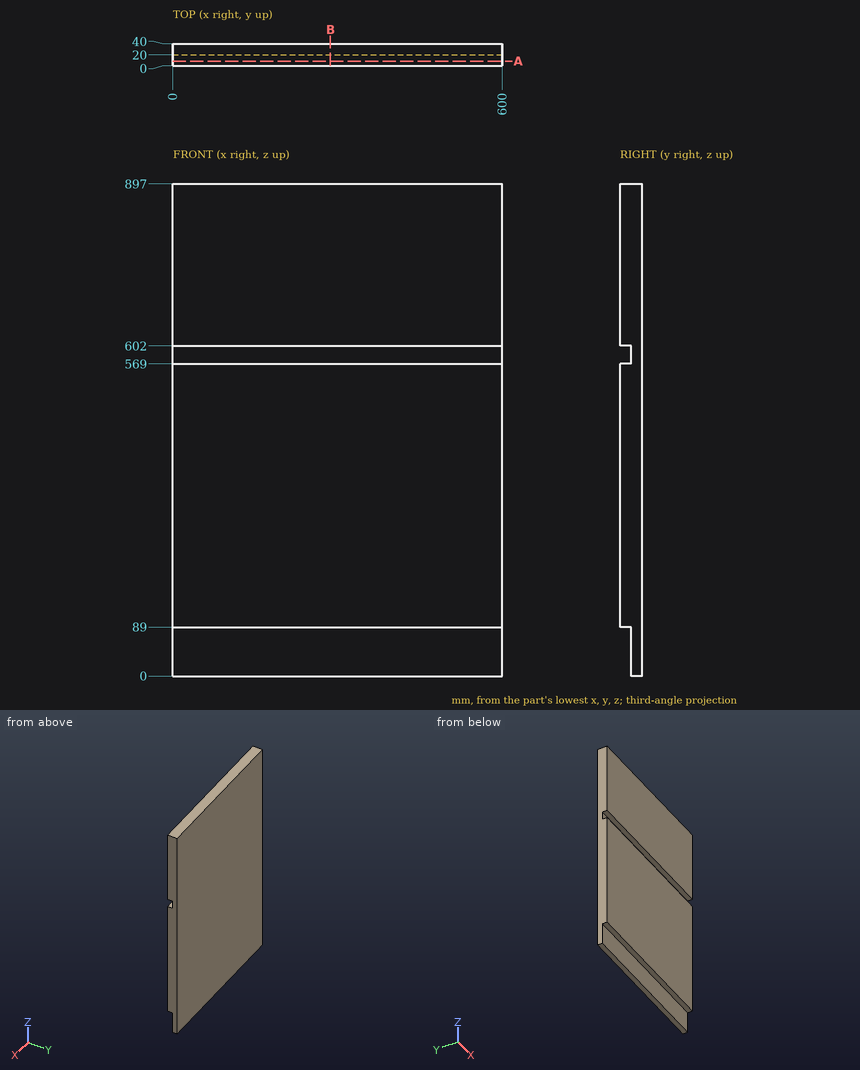
Print and shaded views of the part. All mm, measured from the part's lowest x, y and z. Round coordinates to 2 decimals unless told otherwise and drop trailing zeros. Write each loop counter-clockwise with the first axis right and the second up, starting at its lowest first coordinate (ties: lowest second). Pieces come first, ordered by that corner, then holes.
(1) Slice it at A-A, the plane y = 9. Write the cut outline in (x, z), and give its area (3 significant figures).
(2) Drop a flat-ended pin along its axis: P1, Ø10, axis at x = 443.5, z = 591.5, coming from the -Y side. Give the stop position or say it passes through.
(3) Slice it at B-B, the plane x = 287. Write the cut outline in (y, z).
(4) Probe line 1 along Z through (x, y) = (398.5, 19); line 2 along Y through (x, z) = (218, 83). List the from-to ranges inside material, lowest first.
From the geometry:
1. outline: (0, 89) - (600, 89) - (600, 569) - (0, 569) - close; (0, 602) - (600, 602) - (600, 897) - (0, 897) - close
1. area: 465,000 mm2
2. P1: stops at y = 20
3. outline: (0, 89) - (20, 89) - (20, 0) - (40, 0) - (40, 897) - (0, 897) - (0, 602) - (20, 602) - (20, 569) - (0, 569) - close
4. line 1: z = 89 to 569, 602 to 897
4. line 2: y = 20 to 40
